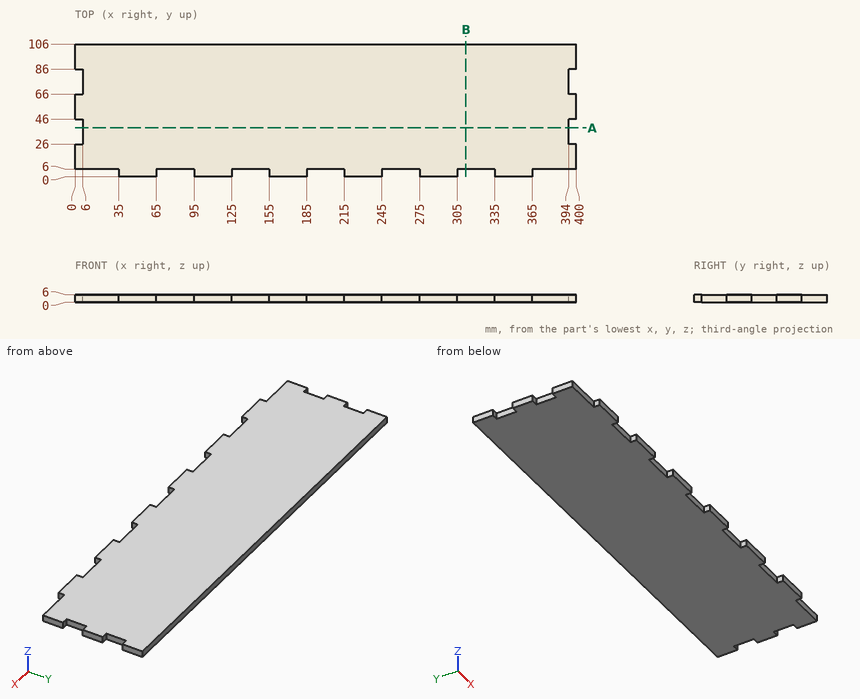
Geometry check sheet. Reference: drawing and pictorial views, mm from the part's lowest x, y, z. Round coordinates to 2 decimals unless told otherwise and drop trailing zeros. Loops run counter-clockwise (first coordinate to the right, second up) from the corner with the lowest first, then second, coordinate; pieces in that order, holes last. Notation, with made-up numbers: (0.5, 28.5) -> (20.5, 28.5) arc R27 ccw to (20.5, 65.5) -> close; hole circle Ø8 at (72.5, 21.5). An arc over 180 degrees is marked (long way). Answer as a JSON object with one key per item and string values. Group by question number.
Item 1: Thickness scan on line 1 along X through (y, z) = (5.5, 1.95); line 2 along X through (y, z) = (35, 5); line 3 along Y through (x, z) = (66, 2.6). Record the ranges inside material, lowest first.
Item 2: Depth check by flat-ended pin: pin 1 Ø1.8 at (y, z) = (4, 3.5) entering from +X; pin 2 Ø3 at (y, z) = (1.5, 4.5) entering from -X; pin 3 Ø3 at (x, z) = (258, 2.5) entering from -Y; pin 4 Ø1 at (x, y) = (185, 71.5) entering from -Z. Enter the tip coordinate at first touch or a pass-through.
Item 3: Cross-section at A-A, the plane y = 39. Record the cut outline in (x, z).
Item 4: Cross-section at B-B, the plane x = 312. Record the cut outline in (y, z).
Determined:
{
 "1": {"line 1": "x = 35 to 65, 95 to 125, 155 to 185, 215 to 245, 275 to 305, 335 to 365", "line 2": "x = 6 to 394", "line 3": "y = 6 to 106"},
 "2": {"pin 1": "stops at x = 365", "pin 2": "stops at x = 35", "pin 3": "stops at y = 6", "pin 4": "stops at z = 0"},
 "3": {"outline": "(6, 0) -> (394, 0) -> (394, 6) -> (6, 6) -> close"},
 "4": {"outline": "(6, 0) -> (106, 0) -> (106, 6) -> (6, 6) -> close"}
}
